Read the model definition and answer for the solid it produces. Units are mm, in the model's axes. Face numbers are marked on the shaded views. A direction names the side the tool comes from. Round coordinates to 2 decimals unless told otherwise and drop trailing zeros. Write each loop counter-clockwise with the first axis right and the second up, starting at its lowest first coordinate (ties: lowest second). Pieces come first, ordered by that corner, then holes. Notation, with made-up numbers: (-5, 88) -> (35, 88) arc R26 cw to (35, 104) -> close; hole circle Ø7 at (89.25, 28.5). An arc over 180 degrees is marked (long way). Return JSON: item names as keys, results as strings. Group by question number.
(1) A cutting plane is placed at C-C on z = 0. Give the vertices of the cut face in (x, y), then the cut area to 3 significant figures.
(2) Given pin 1 (12 mm diameter, centred on y = 69.5, z = 28, fed in from +X); pin 2 (5 mm diameter, centred on y = 28, z = 78, fed in from -X); pin 3 (12 mm diameter, centred on x = 37.5, z = -73.5, fed in from +Y), each flat-ended and moving along its own axis, determine where each tip first touches the part or whether it passes through.
(3) A cutting plane is placed at A-A on y = -5. Give the vertices of the cut face in (x, z).
(4) The mould has two halves that part along X. Classify the marked faces 4, 5 and 6: released by +X, released by -X, zero draft, split by the parting line, or undercut.
(5) A cutting plane is placed at B-B on x = 0. Give the vertices of the cut face in (y, z), then the cut area to 3 significant figures.
(6) For the marked faces 1, 2 and 3, determine the directions among +Z, -Z, +X, -X, +Y, -Y from which every point of the face is accessible in a straight line to the end or side of a thin tool.
(7) A cutting plane is placed at D-D on y = 71. Give the vertices of the cut face in (x, z), then the cut area to 3 significant figures.
(8) Straight lines are drawn through the part: line 1 (X direction, y = 2, z = -10.5); line 2 (Z direction, x = -8, y = -9); line 3 (Y direction, x = -150, z = 44.5). For each, find the intervals that lie inside material, in ascending order.
```python
from build123d import *

# Parameters (mm, degrees)
SKETCH2_R                    = 12
BOSS_EXTRUDE1_DEPTH          = 45
CHAMFER1_SIZE                = 1.5
CIRPATTERN1_COUNT            = 8
CHAMFER1_OF_CIRPATTERN1_SIZE = 1.5


with BuildPart() as part:
    # Sketch1 → Revolve1 (revolve)
    with BuildSketch(Plane.XY, mode=Mode.PRIVATE) as revolve1_sk:
        Polygon((0, 0), (0, 112.5), (30, 112.5), (30, 45), (163.5, 45), (163.5, 7.5), (79.5, 7.5), (79.5, 0), align=None)
    revolve(revolve1_sk.sketch.rotate(Axis((0, 0, 0), (0, 1, 0)), 90), axis=Axis((0, 0, 0), (0, 1, 0)))

    # Sketch2 → Boss-Extrude1 (add)
    with BuildSketch(Plane.XZ.offset(-7.5)):
        with Locations(Location((121.5, 0, 0), (0, 0, 90))):
            Circle(SKETCH2_R)
    boss_extrude1 = extrude(amount=BOSS_EXTRUDE1_DEPTH)

    # Chamfer1
    chamfer1_edges = [part.edges().sort_by_distance(p)[0] for p in [
        (121.5, -37.5, -12),
    ]]
    chamfer(chamfer1_edges, length=CHAMFER1_SIZE)

    # CirPattern1: Boss-Extrude1 ×8 about axis
    cirpattern1_axis = Axis((0, 0, 0), (0, 1, 0))
    for i in range(1, CIRPATTERN1_COUNT):
        add(boss_extrude1.rotate(cirpattern1_axis, i * 360 / CIRPATTERN1_COUNT))

    # Chamfer1 of CirPattern1
    chamfer1_of_cirpattern1_edges = [part.edges().sort_by_distance(p)[0] for p in [
        (77.42819254, -37.5, -94.398755288),
        (-12, -37.5, -121.5),
        (-94.398755288, -37.5, -77.42819254),
        (-121.5, -37.5, 12),
        (-77.42819254, -37.5, 94.398755288),
        (12, -37.5, 121.5),
        (94.398755288, -37.5, 77.42819254),
    ]]
    chamfer(chamfer1_of_cirpattern1_edges, length=CHAMFER1_OF_CIRPATTERN1_SIZE)


solid = part.part
```
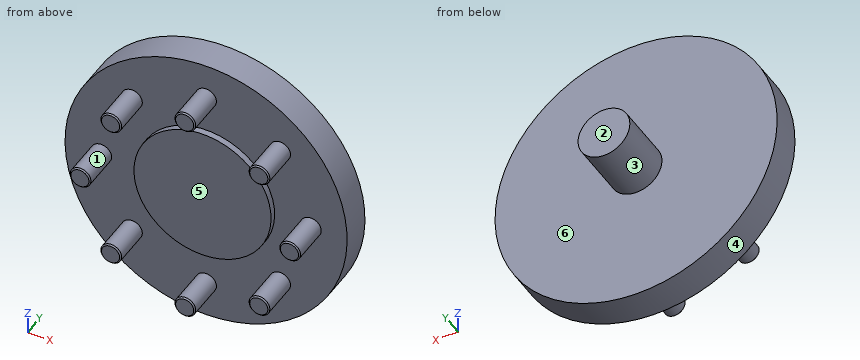
Checks:
{
 "1": {"outline": "(-163.5, 7.5) -> (-133.5, 7.5) -> (-133.5, -36) -> (-132, -37.5) -> (-111, -37.5) -> (-109.5, -36) -> (-109.5, 7.5) -> (-79.5, 7.5) -> (-79.5, 0) -> (79.5, 0) -> (79.5, 7.5) -> (109.5, 7.5) -> (109.5, -36) -> (111, -37.5) -> (132, -37.5) -> (133.5, -36) -> (133.5, 7.5) -> (163.5, 7.5) -> (163.5, 45) -> (30, 45) -> (30, 112.5) -> (-30, 112.5) -> (-30, 45) -> (-163.5, 45) -> close", "area": "19,700 mm^2"},
 "2": {"pin 1": "stops at x = 20.4", "pin 2": "stops at x = -145.02", "pin 3": "stops at y = 45"},
 "3": {"outline": "circle Ø24 at (-121.5, 0); circle Ø24 at (-85.91, -85.91); circle Ø24 at (-85.91, 85.91); circle Ø24 at (0, -121.5); circle Ø24 at (0, 121.5); circle Ø24 at (85.91, -85.91); circle Ø24 at (85.91, 85.91); circle Ø24 at (121.5, 0)"},
 "4": {"face 4": "split by the parting line", "face 5": "undercut", "face 6": "zero draft"},
 "5": {"outline": "(-37.5, -132) -> (-36, -133.5) -> (7.5, -133.5) -> (7.5, -163.5) -> (45, -163.5) -> (45, -30) -> (112.5, -30) -> (112.5, 30) -> (45, 30) -> (45, 163.5) -> (7.5, 163.5) -> (7.5, 133.5) -> (-36, 133.5) -> (-37.5, 132) -> (-37.5, 111) -> (-36, 109.5) -> (7.5, 109.5) -> (7.5, 79.5) -> (0, 79.5) -> (0, -79.5) -> (7.5, -79.5) -> (7.5, -109.5) -> (-36, -109.5) -> (-37.5, -111) -> close", "area": "19,700 mm^2"},
 "6": {"face 1": "-Y", "face 2": "+Z, -Z, +X, -X, +Y", "face 3": "+Y"},
 "7": {"outline": "circle Ø60 at (0, 0)", "area": "2,830 mm^2"},
 "8": {"line 1": "x = -127.31 to -115.69, -78.8 to 78.8, 115.69 to 127.31", "line 2": "z = -130.44 to -112.56, 112.56 to 130.44", "line 3": "y = 7.5 to 45"}
}
